Study the drawing (mm; zero at the part's minimum x, y, z) and answer. Coordinates: 2 decimals unless noted, no trailing zeros. Write each loop counter-clockwise with the first axis right and the second up, starting at its lowest first coordinate (ties: lowest second). Pieces come first, ordered by that corner, then holes. Notation, with made-up numbers: (87.5, 41.5) - (95.5, 41.5) arc R19 ccw to (95.5, 78.5) - close; hole circle Ø10 at (69.25, 30.5). An arc over 180 degrees is marked (long way). One line per item, written item: value.
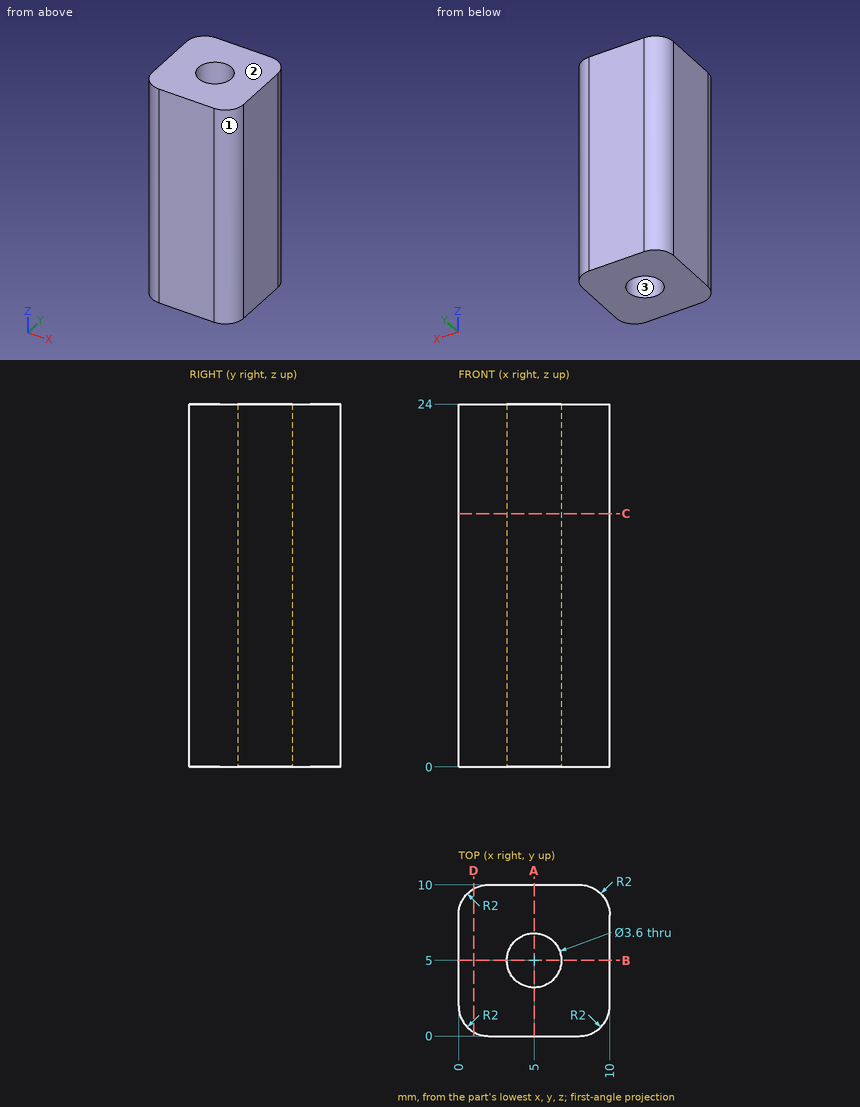
Item 1: Section C-C, the plane z = 16.75 is taken. Determine the outline of the cut face in (x, y), then the cut area to 3 significant figures.
Evaluation:
outline: (0, 2) arc R2 ccw to (2, 0) - (8, 0) arc R2 ccw to (10, 2) - (10, 8) arc R2 ccw to (8, 10) - (2, 10) arc R2 ccw to (0, 8) - close; hole circle Ø3.6 at (5, 5)
area: 86.4 mm2
Item 2: Given pin 1 (1.5 mm diameter, centred on y = 1, z = 11, fed in from +X), flat-ended and moving along its own axis, determine where the tip first touches the part or whether it passes through.
Evaluation:
pin 1: stops at x = 9.98
Item 3: Section A-A, the plane x = 5 is taken. Determine the outline of the cut face in (y, z).
Evaluation:
outline: (0, 0) - (3.2, 0) - (3.2, 24) - (0, 24) - close; (6.8, 0) - (10, 0) - (10, 24) - (6.8, 24) - close
Item 4: Determine the mould class of the marked faces 1, 2 and 3 for opening direction Y: +Y half, -Y half, draft (parallel to the pull), parting line (faces both ways), or undercut.
Evaluation:
face 1: -Y half
face 2: draft
face 3: undercut
Item 5: Section D-D, the plane x = 1 is taken. Determine the outline of the cut face in (y, z).
Evaluation:
outline: (0.27, 0) - (9.73, 0) - (9.73, 24) - (0.27, 24) - close
Item 6: Consider probe 1 along Y at (x, z) = (5, 10.5); probe 2 along Y at (x, z) = (4, 14); probe 3 along X at (y, z) = (6.5, 4.25). Determine where each line is inside the solid, lowest interval first.
Evaluation:
probe 1: y = 0 to 3.2, 6.8 to 10
probe 2: y = 0 to 3.5, 6.5 to 10
probe 3: x = 0 to 4.01, 5.99 to 10
